from build123d import *

# Parameters (mm, degrees)
CUT_EXTRUDE1_DEPTH = 2.5


with BuildPart() as part:
    # Sketch1 → Revolve1 (revolve)
    with BuildSketch(Plane.XY, mode=Mode.PRIVATE) as revolve1_sk:
        Polygon((0, -10), (2.5, -10), (2.5, -2.5), (5, 0), (0, 0), align=None)
    revolve(revolve1_sk.sketch.rotate(Axis((0, 61.691642626, 0), (0, -1, 0)), 90), axis=Axis((0, 61.691642626, 0), (0, -1, 0)))

    # Sketch2 → Cut-Extrude1 (cut)
    with BuildSketch(Plane(origin=(0, 0, 0), x_dir=(-1, 0, 0), z_dir=(0, 1, 0))):
        Polygon((-0.866025404, -1.5), (0.866025404, -1.5), (1.732050808, 0), (0.866025404, 1.5), (-0.866025404, 1.5), (-1.732050808, 0), align=None)
    extrude(amount=-CUT_EXTRUDE1_DEPTH, mode=Mode.SUBTRACT)


solid = part.part
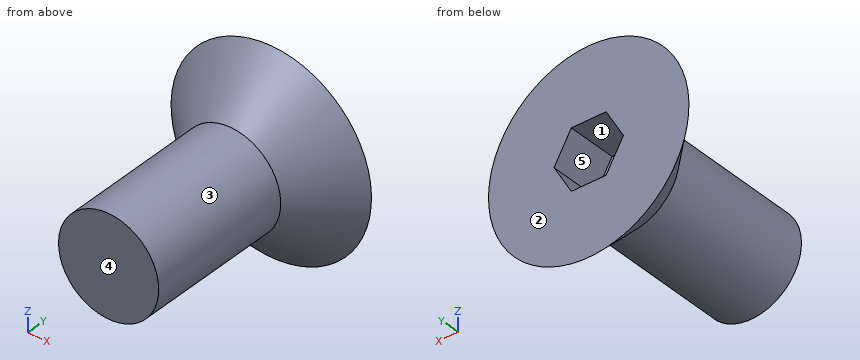
Here's how the part is built. I have some questions about the finished solid (model axes, mm). Face numbers are marked on the shaded views. A direction names the side the tool comes from. Give positions to 0.01 mm unless a question says otherwise; leave off trailing zeros. Order: outer loops, then holes, each group sorted by start corner. A loop starts at its lowest first (then second) coordinate and runs counter-clockwise, first axis right, second up. Notation, with made-up numbers: (87, -35) -> (106, -35) arc R7 cw to (106, -29) -> close; hole circle Ø11 at (85.25, 8.25). An arc over 180 degrees is marked (long way). Use a Markdown table: item, result. Add a question column.
Item 1: I need wall thicknesses on line 1 (Z direction, x = 2, y = -9.5); line 2 (X direction, y = -0.5, z = 1); line 3 (X direction, y = -1.25, z = -0.75). Which ranges of each line are inside material? Lowest first, please.
Item 2: For the marked faces 4 and 5, which set-ups out of +Z, -Z, +X, -X, +Y, -Y let a thin tool reach every point of the face, with its end or its side?
Item 3: Imagine slicing it at A-A on y = -2.25. Please give me the cut outline in (x, z).
Item 4: If we mould it in two halves opening along X, with no side actions, what happens to the marked faces 1, 2 and 3? For each: pulls with the +X half, pulls with the -X half, needs draft (parallel to the pull), parting line crosses it, or undercut.
Item 5: Imagine slicing it at B-B on x = 0. Please give me the cut outline in (y, z).
Item 6: Will these pins go through, and if not, where does the flat tip stop? pin 1 (1 mm diameter, centred on x = -1.5, y = -3, fed in from +Z); pin 2 (0.9 mm diameter, centred on x = 0, y = -1, fed in from +Z); pin 3 (1.5 mm diameter, centred on x = -1.5, y = -4.5, fed in from +Z).
Item 7: Imagine slicing it at C-C on y = -0.25. Please give me the cut outline in (x, z), plus the area to 3 significant figures.
Item 8: Imagine slicing it at D-D on y = -8.25. Please give me the cut outline in (x, z).
Data:
| question | item | result |
|---|---|---|
| 1 | line 1 | z = -1.5 to 1.5 |
| 1 | line 2 | x = -4.39 to -1.15, 1.15 to 4.39 |
| 1 | line 3 | x = -3.67 to -1.3, 1.3 to 3.67 |
| 2 | face 4 | +Z, -Z, +X, -X, -Y |
| 2 | face 5 | +Y |
| 3 | outline | circle Ø5.5 at (0, 0); hole (-1.73, 0) -> (-0.87, -1.5) -> (0.87, -1.5) -> (1.73, 0) -> (0.87, 1.5) -> (-0.87, 1.5) -> close |
| 4 | face 1 | undercut |
| 4 | face 2 | needs draft |
| 4 | face 3 | parting line crosses it |
| 5 | outline | (-10, -2.5) -> (-2.5, -2.5) -> (0, -5) -> (0, -1.5) -> (-2.5, -1.5) -> (-2.5, 1.5) -> (0, 1.5) -> (0, 5) -> (-2.5, 2.5) -> (-10, 2.5) -> close |
| 6 | pin 1 | stops at z = 2.29 |
| 6 | pin 2 | stops at z = 4.45 |
| 6 | pin 3 | stops at z = 2.38 |
| 7 | outline | circle Ø9.5 at (0, 0); hole (-1.73, 0) -> (-0.87, -1.5) -> (0.87, -1.5) -> (1.73, 0) -> (0.87, 1.5) -> (-0.87, 1.5) -> close |
| 7 | area | 63.1 mm² |
| 8 | outline | circle Ø5 at (0, 0) |
